Solid Edge part; units mm, degrees
sketch "Sketch1" plane through (0, 0, 0) normal (0, 0, 1) x (1, 0, 0)
  circle A0 centre (0, 0) radius 1.621
  circle A1 centre (0, 0) radius 4.0415
extrude "Protrusion1" add sketch "Sketch1" along normal blind 4.2
sketch "Sketch2" plane through (0, 0, 0) normal (0, 0, 1) x (1, 0, 0)
  line L0 (4.0415, 0) -> (2.0207, 3.5)
  arc A0 (2.0207, 3.5) -> (4.0415, 0) centre (0, 0) cw
extrude "ExtrudedCutout_1" cut sketch "Sketch2" along normal blind 4.2
pattern_circular "Pattern1" count 6 over 360 about axis through (0, 0, 0) along (0, 0, -1) of "ExtrudedCutout_1"
cosmetic_thread "Thread_1" thread depth 2.7
sketch "Sketch3" plane through (0, 0, 0) normal (0, -1, 0) x (1, 0, 0)
  line L0 (4.0416, 0.3199) -> (4.0416, 0)
  line L1 (4.0416, 0) -> (3.4875, 0)
  line L2 (3.4875, 0) -> (4.0416, 0.3199)
  line L3 (3.3, 4.2) -> (3.3, 2.9309)
  arc A0 (3.3, 2.9309) -> (3.5, 2.5845) centre (3.7, 2.9309) ccw
  line L4 (3.5, 2.5845) -> (4.0416, 2.2718)
  line L5 (4.0416, 2.2718) -> (4.0416, 4.2)
  line L6 (4.0416, 4.2) -> (3.3, 4.2)
  dimension "D1" = 3.3
revolve "RevolvedCutout_1" cut sketch "Sketch3" angle 360 about axis through (0, 0, 11.9) along (0, 0, -1)
sketch "Sketch4" plane through (0, 0, 0) normal (0, -1, 0) x (1, 0, 0)
  line L0 (1.621, 4.2) -> (1.621, 2.7)
  line L1 (2.15, 4.2) -> (1.621, 4.2)
  line L2 (2.15, 3.8) -> (2.15, 4.2)
  line L3 (1.646, 3.8) -> (2.15, 3.8)
  line L4 (1.646, 3.8) -> (1.646, 2.7)
  line L5 (1.646, 2.7) -> (1.621, 2.7)
  dimension "D1" = 2.15
  dimension "D2" = 1.621
  dimension "D3" = 1.646
revolve "RevolvedCutout_2" cut sketch "Sketch4" angle 360 about axis through (0, 0, 8.4) along (0, 0, -1)
fillet "Round_1" radius 0.3 2 edges at (-3.3, 0, 4.2) (-2.15, 0, 4.2)
chamfer "Chamfer_1" distance 0.679 angle 30 1 edges at (-1.621, 0, 0) measured on face at (-2.3947, -2.2552, 0)
properties material "Stahl"
Part model, mm, in its own coordinate system. A direction names the side the tool comes from. Coordinates: 2 decimals unless noted, no trailing zeros. Order: outer loops, then holes, each group sorted by start corner. A loop starts at its lowest first (then second) coordinate and runs counter-clockwise, first axis right, second up. Notation, with made-up numbers: (41.5, 76.5) - (73.5, 76.5) arc R15 cw to (73.5, 81.5) - close; hole circle Ø10 at (35, 19). An arc over 180 degrees is marked (long way). Return JSON: item names as keys, results as strings. Group by question number.
Item 1: Drill centre lines: probe 1 along Y at (x, z) = (0, 1.85); probe 2 along X at (y, z) = (0, 3.05); probe 3 along Y at (x, z) = (0, 3.85). Where is each one in solid material? Low to high. Write a range as from..to.
Item 2: Pull direction X, two halves, no side cores. Call faces 3 (the face through (3, -1.8, 1.3)), 4 (the face through (-3.632, -0.009, 2.508)), 5 (the face through (0.748, 1.438, 1.53)): pulls with the +X half, pulls with the -X half, needs draft (parallel to the pull), parting line crosses it, or undercut.
Item 3: Cut at B-B (z = 3.6). List the corners of the cut face in (x, y).
Item 4: Which spindle directions (+Z, -Z, +X, -X, +Y, -Y) get a long thin tool onto all of the face, cutting with end or side? Do faces 1 (the face through (-2.43, -2.23, 3.41)), 2 (the face through (3.045, 1.725, 1.278)). Say none if no direction does.
Item 5: Pin check, flat tip, straight feed: pin 1 (4 mm diameter, centred on x = 0, y = 0, fed in from +Z). Stop position of the tip, or through.
Item 6: Cut at A-A (z = 1.35). List the corners of the cut face in (x, y), plus the area to 3 significant figures.
Check values:
{
 "1": {"probe 1": "y = -3.5..-1.62, 1.62..3.5", "probe 2": "x = -3.3..-1.65, 1.65..3.3", "probe 3": "y = -3.3..-2.15, 2.15..3.3"},
 "2": {"face 3": "pulls with the +X half", "face 4": "pulls with the -X half", "face 5": "undercut"},
 "3": {"outline": "circle Ø6.6 at (0, 0); hole circle Ø3.29 at (0, 0)"},
 "4": {"face 1": "+Z", "face 2": "+Z, -Z, +X, +Y"},
 "5": {"pin 1": "stops at z = 3.8"},
 "6": {"outline": "(-4.04, 0) - (-2.02, -3.5) - (2.02, -3.5) - (4.04, 0) - (2.02, 3.5) - (-2.02, 3.5) - close; hole circle Ø3.24 at (0, 0)", "area": "34.2 mm2"}
}
